The model under review builds one solid part; all positions refer to its coordinate system, in mm. Face numbers are marked on the shaded views. A direction names the side the tool comes from. Coordinates: 2 decimals unless noted, no trailing zeros. Write each loop counter-clockwise with the first axis right and the second up, starting at its lowest first coordinate (ties: lowest second). Pieces come first, ordered by that corner, then holes. Notation, with made-up numbers: (-28, -25.5) - (-2, -25.5) arc R20 ccw to (-2, -4.5) - close; hole circle Ø9 at (-38.75, 50.5). An arc over 180 degrees is marked (long way). Put each result on its own line as item: value.
Autodesk Fusion 360 part; units mm, degrees
sketch "Sketch1" plane through (0, 0, 0) normal (0, 0, 1) x (1, 0, 0)
  line L0 (0, 0) -> (0, 6)
  line L1 (0, 6) -> (6, 6)
  line L2 (6, 6) -> (6, 0)
  line L3 (6, 0) -> (0, 0)
  dimension "d1" = 6
  dimension "d2" = 6
extrude "Extrude1" add sketch "Sketch1" along normal blind 13.75
sketch "Sketch2" plane through (0, 0, 13.75) normal (0, 0, 1) x (-1, 0, 0)
  line L0 (-6, 0) -> (-6, -6)
  line L1 (-6, -6) -> (0, -6)
  line L2 (0, -6) -> (0, 0)
  line L3 (0, 0) -> (-6, 0)
  circle A0 centre (-3, -3) radius 1.2
  dimension "d6" = 2.4
extrude "Extrude2" add sketch "Sketch2" along normal blind 2 contours A0
sketch "Sketch3" plane through (0, 0, 0) normal (0, 0, -1) x (1, 0, 0)
  line L0 (6, -6) -> (6, 0)
  line L1 (6, 0) -> (0, 0)
  line L2 (0, 0) -> (0, -6)
  line L3 (0, -6) -> (6, -6)
  circle A0 centre (3, -3) radius 1.4
  dimension "d9" = 2.8
extrude "Extrude3" cut sketch "Sketch3" against normal blind 12 contours A0
fillet "Fillet1" radius 0.8 4 edges at (6, 0, 6.875) (6, 6, 6.875) (0, 6, 6.875) (0, 0, 6.875)
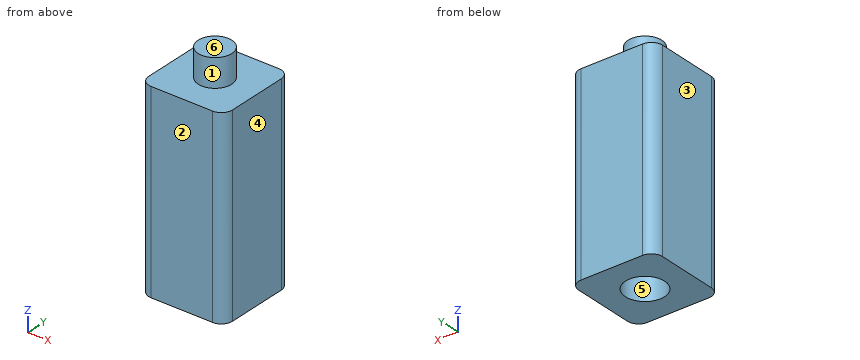
1. The part is to be moulded in two halves that separate along X. For the marked faces 3, 4, 5 and 6, say which applies: +X half, -X half, draft (parallel to the pull), parting line (faces both ways), or undercut.
Determined:
face 3: -X half
face 4: +X half
face 5: undercut
face 6: draft
2. Consider section A-A on y = 3. State the section outline as (x, z) points.
Determined:
outline: (0, 0) - (1.6, 0) - (1.6, 12) - (4.4, 12) - (4.4, 0) - (6, 0) - (6, 13.75) - (4.2, 13.75) - (4.2, 15.75) - (1.8, 15.75) - (1.8, 13.75) - (0, 13.75) - close
3. For pin 1 Ø0.8 at (x, y) = (3.5, 3.5) entering from -Z, flat-tipped, find the tip position at first contact; note if it passes through.
Determined:
pin 1: stops at z = 12
4. To check wall thickness, follow probe 1 along X at (y, z) = (3, 4.5); probe 2 along Z at (x, y) = (1.6, 2.6). State the ranges of each line that lie inside material, in increasing order.
Determined:
probe 1: x = 0 to 1.6, 4.4 to 6
probe 2: z = 0 to 13.75
5. Consider section B-B on z = 11.25. State the section outline as (x, y) points, plus the area to 3 significant figures.
Determined:
outline: (0, 0.8) arc R0.8 ccw to (0.8, 0) - (5.2, 0) arc R0.8 ccw to (6, 0.8) - (6, 5.2) arc R0.8 ccw to (5.2, 6) - (0.8, 6) arc R0.8 ccw to (0, 5.2) - close; hole circle Ø2.8 at (3, 3)
area: 29.3 mm^2
6. Consider section D-D on y = 1.15. State the section outline as (x, z) points.
Determined:
outline: (0, 0) - (6, 0) - (6, 13.75) - (0, 13.75) - close
7. Machinability: for the marked faces 1 and 2, which of the approach directions +Z, -Z, +X, -X, +Y, -Y give a long, thin tool a straight path to every point of the face, cutting with its end or side? Answer none if there is none.
Determined:
face 1: +Z
face 2: +Z, -Z, +X, -X, -Y
